Work out the finished part from the listing and answer in its coordinate system (mm). Face numbers are marked on the shaded views. A direction names the side the tool comes from. Give positions to 0.01 mm unless a question says otherwise; leave off trailing zeros. Loops run counter-clockwise (first coordinate to the right, second up) from the corner with the lowest first, then second, coordinate; pieces in that order, holes last. Notation, with made-up numbers: (38.5, -27) - (67.5, -27) arc R35 cw to (67.5, 9) - close; hole circle Ø3 at (-35.5, 15.25). An arc over 180 degrees is marked (long way). Use CSV: the item, a comma, the result in double quotes.
from build123d import *

# Parameters (mm, degrees)
SKETCH1_R           = 2.1
BOSS_EXTRUDE1_DEPTH = 8
SKETCH2_R           = 2.1
CUT_EXTRUDE1_DEPTH  = 5.8


with BuildPart() as part:
    # Sketch1 → Boss-Extrude1 (new body)
    with BuildSketch(Plane(origin=(0, 0, 0), x_dir=(1, 0, 0), z_dir=(0, 1, 0))):
        with BuildLine():
            Line((-4, -22), (-4, -17.549928775))
            ThreePointArc((-4, -17.549928775), (-15.588457268, -9), (-17.198684154, 5.310862772))
            Line((-17.198684154, 5.310862772), (-21.052558883, 7.535898385))
            ThreePointArc((-21.052558883, 7.535898385), (-22.516660498, 13), (-17.052558883, 14.464101615))
            Line((-17.052558883, 14.464101615), (-13.198684154, 12.239066003))
            ThreePointArc((-13.198684154, 12.239066003), (0, 18), (13.198684154, 12.239066003))
            Line((13.198684154, 12.239066003), (17.052558883, 14.464101615))
            ThreePointArc((17.052558883, 14.464101615), (22.516660498, 13), (21.052558883, 7.535898385))
            Line((21.052558883, 7.535898385), (17.198684154, 5.310862772))
            ThreePointArc((17.198684154, 5.310862772), (15.588457268, -9), (4, -17.549928775))
            Line((4, -17.549928775), (4, -22))
            ThreePointArc((4, -22), (0, -26), (-4, -22))
        make_face()
        with Locations((0, -22)):
            Circle(SKETCH1_R, mode=Mode.SUBTRACT)
        with Locations((-19.052558883, 11)):
            Circle(SKETCH1_R, mode=Mode.SUBTRACT)
        with Locations((19.052558883, 11)):
            Circle(SKETCH1_R, mode=Mode.SUBTRACT)
        with BuildLine():
            Line((1, 4.898979486), (1, 14))
            ThreePointArc((1, 14), (0, 15), (-1, 14))
            Line((-1, 14), (-1, 4.898979486))
            ThreePointArc((-1, 4.898979486), (-2.5, 4.330127019), (-3.742640687, 3.315515147))
            Line((-3.742640687, 3.315515147), (-11.624355653, 7.866025404))
            ThreePointArc((-11.624355653, 7.866025404), (-12.990381057, 7.5), (-12.624355653, 6.133974596))
            Line((-12.624355653, 6.133974596), (-4.742640687, 1.583464339))
            ThreePointArc((-4.742640687, 1.583464339), (-5, 0), (-4.742640687, -1.583464339))
            Line((-4.742640687, -1.583464339), (-12.624355653, -6.133974596))
            ThreePointArc((-12.624355653, -6.133974596), (-12.990381057, -7.5), (-11.624355653, -7.866025404))
            Line((-11.624355653, -7.866025404), (-3.742640687, -3.315515147))
            ThreePointArc((-3.742640687, -3.315515147), (-2.5, -4.330127019), (-1, -4.898979486))
            Line((-1, -4.898979486), (-1, -14))
            ThreePointArc((-1, -14), (0, -15), (1, -14))
            Line((1, -14), (1, -4.898979486))
            ThreePointArc((1, -4.898979486), (2.5, -4.330127019), (3.742640687, -3.315515147))
            Line((3.742640687, -3.315515147), (11.624355653, -7.866025404))
            ThreePointArc((11.624355653, -7.866025404), (12.990381057, -7.5), (12.624355653, -6.133974596))
            Line((12.624355653, -6.133974596), (4.742640687, -1.583464339))
            ThreePointArc((4.742640687, -1.583464339), (5, 0), (4.742640687, 1.583464339))
            Line((4.742640687, 1.583464339), (12.624355653, 6.133974596))
            ThreePointArc((12.624355653, 6.133974596), (12.990381057, 7.5), (11.624355653, 7.866025404))
            Line((11.624355653, 7.866025404), (3.742640687, 3.315515147))
            ThreePointArc((3.742640687, 3.315515147), (2.5, 4.330127019), (1, 4.898979486))
        make_face(mode=Mode.SUBTRACT)
    extrude(amount=BOSS_EXTRUDE1_DEPTH)

    # Sketch2 → Cut-Extrude1 (cut)
    with BuildSketch(Plane(origin=(0, 8, 0), x_dir=(1, 0, 0), z_dir=(0, 1, 0))):
        with Locations((10, 0)):
            Circle(SKETCH2_R)
        with Locations((5, -8.660254038)):
            Circle(SKETCH2_R)
        with Locations((-5, -8.660254038)):
            Circle(SKETCH2_R)
        with Locations((-10, 0)):
            Circle(SKETCH2_R)
        with Locations((-5, 8.660254038)):
            Circle(SKETCH2_R)
        with Locations((5, 8.660254038)):
            Circle(SKETCH2_R)
    extrude(amount=-CUT_EXTRUDE1_DEPTH, mode=Mode.SUBTRACT)


solid = part.part
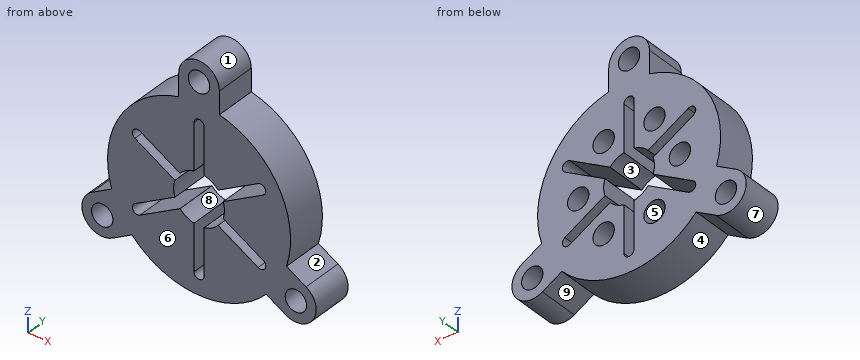
Item 1: A cutting plane is placed at A-A on z = 0. Determine the outline of the cut face in (x, y), and give its area (3 significant figures).
Determined:
outline,"(-18, 0) - (-5, 0) - (-5, 8) - (-7.9, 8) - (-7.9, 2.2) - (-12.1, 2.2) - (-12.1, 8) - (-18, 8) - close; (5, 0) - (18, 0) - (18, 8) - (12.1, 8) - (12.1, 2.2) - (7.9, 2.2) - (7.9, 8) - (5, 8) - close"
area,"159 mm²"
Item 2: Given P1, Ø3, axis at y = 6.5, z = 20, coming from the -X side; P2, Ø4, axis at x = -10, z = 0, coming from the +Y side; P3, Ø2, axis at y = 3, z = 20.5, coming from the +X side, each flat-ended and moving along its own axis, determine where each tip first touches the part or whether it passes through.
Determined:
P1,"stops at x = -4"
P2,"stops at y = 2.2"
P3,"stops at x = 4"
Item 3: The mould has two halves that part along Z. Classify the marked faces 6, 7, 8 and 9: pulls with the +Z half, pulls with the -Z half, needs draft (parallel to the pull), parting line crosses it, or undercut.
Determined:
face 6,"needs draft"
face 7,"parting line crosses it"
face 8,"undercut"
face 9,"pulls with the -Z half"
Item 4: A cutting plane is placed at D-D on z = 10. Determine the outline of the cut face in (x, y).
Determined:
outline,"(-14.97, 0) - (-1, 0) - (-1, 8) - (-3.38, 8) - (-3.38, 2.2) - (-6.62, 2.2) - (-6.62, 8) - (-14.97, 8) - close; (1, 0) - (14.97, 0) - (14.97, 8) - (6.62, 8) - (6.62, 2.2) - (3.38, 2.2) - (3.38, 8) - (1, 8) - close"
Item 5: A cutting plane is placed at B-B on x = 11. Determine the outline of the cut face in (y, z).
Determined:
outline,"(0, -14.25) - (8, -14.25) - (8, -7.51) - (0, -7.51) - close; (0, -5.2) - (8, -5.2) - (8, -1.85) - (2.2, -1.85) - (2.2, 1.85) - (8, 1.85) - (8, 5.2) - (0, 5.2) - close; (0, 7.51) - (8, 7.51) - (8, 14.25) - (0, 14.25) - close"
Item 6: For the marked faces 1, 2, 3, 4 and 5, determine the directions among +Z, -Z, +X, -X, +Y, -Y from which every point of the face is accessible in a straight line to the end or side of a thin tool.
Determined:
face 1,"+Z, +Y, -Y"
face 2,"+X, +Y, -Y"
face 3,"+Y, -Y"
face 4,"-Z, +Y, -Y"
face 5,"+Y"
Item 7: Find the intervals of material crossed by line 1 (Z direction, x = 10, y = 6.4); line 2 (X direction, y = 3.5, z = -10); line 3 (X direction, y = 7, z = 8.5), in increasing order.
Determined:
line 1,"z = -14.97 to -6.93, -4.62 to -2.1, 2.1 to 4.62, 6.93 to 14.97"
line 2,"x = -22.93 to -20.9, -17.21 to -6.62, -3.38 to -1, 1 to 3.38, 6.62 to 17.21, 20.9 to 22.93"
line 3,"x = -15.87 to -7.09, -2.91 to -1, 1 to 2.91, 7.09 to 15.87"
Item 8: A cutting plane is placed at C-C on y = 1.5. State how many separate pieces and enclosed holes the cut face has, and give its area (3 significant figures).
Determined:
separate pieces,"1"
enclosed holes,"4"
area,"955 mm²"
